For this review, take the finished solid that the model builds, in its own axes (mm). Face numbers are marked on the shaded views. A direction names the side the tool comes from. Round coordinates to 2 decimals unless told otherwise and drop trailing zeros. Write each loop counter-clockwise with the first axis right and the second up, starting at its lowest first coordinate (ties: lowest second). Pieces come first, ordered by that corner, then holes. Notation, with made-up numbers: (63.25, -34.5) -> (77.25, -34.5) arc R21 cw to (77.25, -12.5) -> close; hole circle Ø1 at (-20, 42.25). An arc over 180 degrees is marked (long way). Answer in a Markdown table with one row per item. Add a question column.
```python
from build123d import *

# Parameters (mm, degrees)
BASE_DEPTH          = 10
BASE_DEPTH_BACK     = 10
ESQUISSE1_R         = 25
ESQUISSE2_R         = 25
ESQUISSE2_R_2       = 23
VIDE_GORGE_DEPTH    = 7
VIDE_JANTE_DEPTH    = 20
ESQUISSE6_R         = 3
VIDE_BLOC_AXE_DEPTH = 4


with BuildPart() as part:
    # Esquisse1 → BASE (new, two sides: drawn at the far end of the back side and taken through both)
    with BuildSketch(Plane(origin=(0, 0, 0), x_dir=(0, 0, -1), z_dir=(1, 0, 0)).offset(-BASE_DEPTH_BACK)):
        Circle(ESQUISSE1_R)
        with BuildLine():
            Line((-1.658312395, 2.5), (1.658312395, 2.5))
            ThreePointArc((1.658312395, 2.5), (0, -3), (-1.658312395, 2.5))
        make_face(mode=Mode.SUBTRACT)
    extrude(amount=BASE_DEPTH + BASE_DEPTH_BACK)

    # Esquisse2 → VIDE GORGE (cut)
    with BuildSketch(Plane.ZY.offset(8)):
        with Locations(Location((0, 0, 0), (0, 0, 180))):
            Circle(ESQUISSE2_R)
        Circle(ESQUISSE2_R_2, mode=Mode.SUBTRACT)
    vide_gorge = extrude(amount=-VIDE_GORGE_DEPTH, mode=Mode.SUBTRACT)

    # SYM GORGE: VIDE GORGE across plane
    add(vide_gorge.mirror(Plane(origin=(0, 0, 0), x_dir=(0, 0, 1), z_dir=(1, 0, 0))), mode=Mode.SUBTRACT)

    # Esquisse4 → VIDE JANTE (cut)
    with BuildSketch(Plane(origin=(10, 0, 0), x_dir=(0, 0, -1), z_dir=(1, 0, 0))):
        with BuildLine():
            Line((-22, 0), (-5, 0))
            ThreePointArc((-5, 0), (-4.924038765, 0.868240888), (-4.698463104, 1.710100717))
            Line((-4.698463104, 1.710100717), (-20.673237657, 7.524443153))
            ThreePointArc((-20.673237657, 7.524443153), (-21.665770566, 3.820259909), (-22, 0))
        make_face()
        with BuildLine():
            ThreePointArc((-4.698463104, -1.710100717), (-4.924038765, -0.868240888), (-5, 0))
            Line((-5, 0), (-22, 0))
            ThreePointArc((-22, 0), (-21.665770566, -3.820259909), (-20.673237657, -7.524443153))
            Line((-20.673237657, -7.524443153), (-4.698463104, -1.710100717))
        make_face()
        with BuildLine():
            Line((-13.544552457, 17.336236579), (-3.078307377, 3.940053768))
            ThreePointArc((-3.078307377, 3.940053768), (-1.545084972, 4.755282581), (0.174497484, 4.996954135))
            Line((0.174497484, 4.996954135), (0.767788927, 21.986598194))
            ThreePointArc((0.767788927, 21.986598194), (-6.798373876, 20.923243358), (-13.544552457, 17.336236579))
        make_face()
        with BuildLine():
            Line((12.302243876, 18.238826596), (2.795964517, 4.145187863))
            ThreePointArc((2.795964517, 4.145187863), (4.045084972, 2.938926261), (4.80630848, 1.378186779))
            Line((4.80630848, 1.378186779), (21.147757311, 6.064021828))
            ThreePointArc((21.147757311, 6.064021828), (17.798373876, 12.93127555), (12.302243876, 18.238826596))
        make_face()
        with BuildLine():
            ThreePointArc((4.80630848, -1.378186779), (4.045084972, -2.938926261), (2.795964517, -4.145187863))
            Line((2.795964517, -4.145187863), (12.302243876, -18.238826596))
            ThreePointArc((12.302243876, -18.238826596), (17.798373876, -12.93127555), (21.147757311, -6.064021828))
            Line((21.147757311, -6.064021828), (4.80630848, -1.378186779))
        make_face()
        with BuildLine():
            ThreePointArc((0.174497484, -4.996954135), (-1.545084972, -4.755282581), (-3.078307377, -3.940053768))
            Line((-3.078307377, -3.940053768), (-13.544552457, -17.336236579))
            ThreePointArc((-13.544552457, -17.336236579), (-6.798373876, -20.923243358), (0.767788927, -21.986598194))
            Line((0.767788927, -21.986598194), (0.174497484, -4.996954135))
        make_face()
    extrude(amount=-VIDE_JANTE_DEPTH, mode=Mode.SUBTRACT)

    # Esquisse6 → VIDE BLOC AXE (cut)
    with BuildSketch(Plane.ZY.offset(10)):
        with Locations(Location((0, 0, 0), (0, 0, 180))):
            Circle(ESQUISSE6_R)
    extrude(amount=-VIDE_BLOC_AXE_DEPTH, mode=Mode.SUBTRACT)


solid = part.part
```
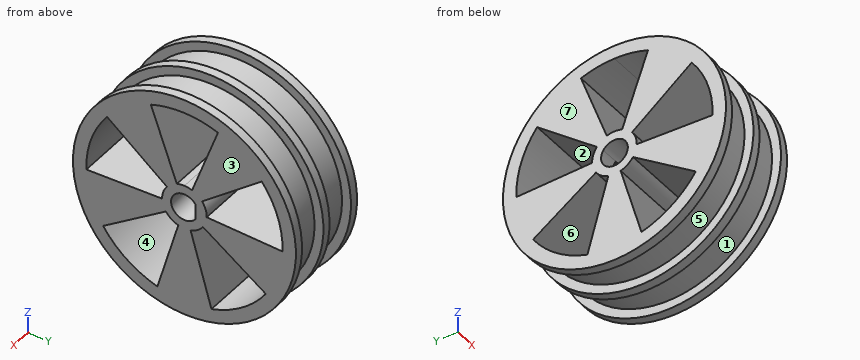
1. Tool access review of the marked faces 5, 6 and 7: name each direction out of +Z, -Z, +X, -X, +Y, -Y from which nothing blocks a thin tool from reaching the whole face with its end or side.
2. We need section A-A (x = 5). Write out the cut boundary in (y, z), plus the area to 3 significant figures.
3. For L1, parallel to Y at x = -4, z = 0; L2, parallel to Y at x = -0.75, z = 0; L3, parallel to Z at x = 1.75, y = 14.5, list the stretches that pass through material, from the lowest coordinate up. Write a range as [from, to].
4. We need section B-B (y = 11.5). Write out the cut boundary in (x, z) (3 decimals), plus the area to 3 significant figures.
5. Clearance check with flat-ended pins moving along their axes: pin 1 Ø3 at (x, y) = (-4, -16) entering from -Z; pin 2 Ø8 at (x, z) = (2.5, -1) entering from -Y; pin 3 Ø1.5 at (x, z) = (6.5, -18.5) entering from +Y; pin 4 Ø15 at (y, z) = (-0.5, 11) entering from +X. State where each tip first meets the part, or that it passes through.
6. The part is to be moulded in two halves that separate along Z. For the marked faces 1, 2, 3 and 4, say which applies: pulls with the +Z half, pulls with the -Z half, needs draft (parallel to the pull), parting line crosses it, or undercut.
7. We need section C-C (z = -13). Write out the cut boundary in (x, y).
Response:
| question | item | result |
|---|---|---|
| 1 | face 5 | none |
| 1 | face 6 | +X, -X |
| 1 | face 7 | +Z, -Z, -X, +Y, -Y |
| 2 | outline | circle Ø46 at (0, 0); hole (-21.99, -0.77) -> (-5, -0.17) arc R5 cw to (-3.94, 3.08) -> (-17.34, 13.54) arc R22 ccw to start; hole (-18.24, -12.3) arc R22 ccw to (-6.06, -21.15) -> (-1.38, -4.81) arc R5 cw to (-4.15, -2.8) -> close; hole (-7.52, 20.67) -> (-1.71, 4.7) arc R5 cw to (1.71, 4.7) -> (7.52, 20.67) arc R22 ccw to start; hole (1.38, -4.81) -> (6.06, -21.15) arc R22 ccw to (18.24, -12.3) -> (4.15, -2.8) arc R5 cw to start; hole (2.5, -1.66) -> (2.5, 1.66) arc R3 ccw (long way) to start; hole (3.94, 3.08) arc R5 cw to (5, -0.17) -> (21.99, -0.77) arc R22 ccw to (17.34, 13.54) -> close |
| 2 | area | 834 mm2 |
| 3 | L1 | [-23, -22], [-5, -3], [2.5, 5], [22, 23] |
| 3 | L2 | [-25, -22], [-5, -3], [2.5, 5], [22, 25] |
| 3 | L3 | [-17.85, -16.55], [-9.78, -0.51], [11.33, 17.85] |
| 4 | outline | (-10, -22.198) -> (-8, -22.198) -> (-8, -19.919) -> (-1, -19.919) -> (-1, -22.198) -> (1, -22.198) -> (1, -19.919) -> (8, -19.919) -> (8, -22.198) -> (10, -22.198) -> (10, -18.755) -> (-10, -18.755) -> close; (-10, -7.757) -> (10, -7.757) -> (10, -0.402) -> (-10, -0.402) -> close; (-10, 8.985) -> (10, 8.985) -> (10, 22.198) -> (8, 22.198) -> (8, 19.919) -> (1, 19.919) -> (1, 22.198) -> (-1, 22.198) -> (-1, 19.919) -> (-8, 19.919) -> (-8, 22.198) -> (-10, 22.198) -> close |
| 4 | area | 416 mm2 |
| 5 | pin 1 | z = -17.85 |
| 5 | pin 2 | y = -25 |
| 5 | pin 3 | y = 14.63 |
| 5 | pin 4 | x = 10 |
| 6 | face 1 | parting line crosses it |
| 6 | face 2 | undercut |
| 6 | face 3 | needs draft |
| 6 | face 4 | undercut |
| 7 | outline | (-10, -21.35) -> (-8, -21.35) -> (-8, -18.97) -> (-1, -18.97) -> (-1, -21.35) -> (1, -21.35) -> (1, -18.97) -> (8, -18.97) -> (8, -21.35) -> (10, -21.35) -> (10, -17.75) -> (-10, -17.75) -> close; (-10, -3.73) -> (10, -3.73) -> (10, 3.73) -> (-10, 3.73) -> close; (-10, 17.75) -> (10, 17.75) -> (10, 21.35) -> (8, 21.35) -> (8, 18.97) -> (1, 18.97) -> (1, 21.35) -> (-1, 21.35) -> (-1, 18.97) -> (-8, 18.97) -> (-8, 21.35) -> (-10, 21.35) -> close |
